```python
from build123d import *

# Parameters (mm, degrees)
SKETCH1_W                 = 75
SKETCH1_H                 = 40
BOSS_EXTRUDE1_DEPTH       = 8
SKETCH2_W                 = 72
SKETCH2_H                 = 17
SKETCH2_W_2               = 71
SKETCH2_H_2               = 16
CUT_EXTRUDE1_DEPTH        = 0.5
SKETCH3_W                 = 15
SKETCH3_H                 = 5
SKETCH3_W_2               = 7
SKETCH3_H_2               = 7
CUT_EXTRUDE3_DEPTH        = 3
DRAFT4_ANGLE              = 25
DRAFT5_ANGLE              = 25
DRAFT4_OF_MIRROR1_2_ANGLE = 25
DRAFT5_OF_MIRROR1_2_ANGLE = 25


with BuildPart() as part:
    # Sketch1 → Boss-Extrude1 (new body)
    with BuildSketch(Plane.XY):
        with Locations((37.5, 20)):
            Rectangle(SKETCH1_W, SKETCH1_H)
    extrude(amount=BOSS_EXTRUDE1_DEPTH)

    # Sketch2 → Cut-Extrude1 (cut)
    with BuildSketch(Plane.XY.offset(8)):
        with Locations((37.5, 10)):
            Rectangle(SKETCH2_W, SKETCH2_H)
        with Locations((37.5, 10)):
            Rectangle(SKETCH2_W_2, SKETCH2_H_2, mode=Mode.SUBTRACT)
    cut_extrude1 = extrude(amount=-CUT_EXTRUDE1_DEPTH, mode=Mode.SUBTRACT)

    # Sketch3 → Cut-Extrude3 (cut)
    with BuildSketch(Plane.XY.offset(8)):
        with Locations((37.5, 10)):
            Rectangle(SKETCH3_W, SKETCH3_H)
        with Locations((63.5, 10)):
            Rectangle(SKETCH3_W_2, SKETCH3_H_2)
    cut_extrude3 = extrude(amount=-CUT_EXTRUDE3_DEPTH, mode=Mode.SUBTRACT)

    # Draft4
    draft4_faces = [part.faces().sort_by_distance(p)[0] for p in [
        (45, 10, 6.5),
        (37.5, 7.5, 6.5),
        (30, 10, 6.5),
        (37.5, 12.5, 6.5),
    ]]
    draft(draft4_faces, Plane.XY.offset(8), DRAFT4_ANGLE)

    # Draft5
    draft5_faces = [part.faces().sort_by_distance(p)[0] for p in [
        (67, 10, 6.5),
        (63.5, 6.5, 6.5),
        (60, 10, 6.5),
        (63.5, 13.5, 6.5),
    ]]
    draft(draft5_faces, Plane.XY.offset(8), DRAFT5_ANGLE)

    # Sketch7 → Revolve2 (revolve)
    with BuildSketch(Plane(origin=(63.5, 0, 0), x_dir=(0, 0, -1), z_dir=(1, 0, 0)), mode=Mode.PRIVATE) as revolve2_sk:
        Polygon((-5, 10), (-5, 9.5), (-6.936491673, 10), align=None)
    revolve2 = revolve(revolve2_sk.sketch.rotate(Axis((63.5, 10, 6.936491673), (0, 0, -1)), 90), axis=Axis((63.5, 10, 6.936491673), (0, 0, -1)))

    # Mirror1: Cut-Extrude1, Cut-Extrude3, Revolve2 across plane
    add(cut_extrude1.mirror(Plane.ZX.offset(20)), mode=Mode.SUBTRACT)
    add(cut_extrude3.mirror(Plane.ZX.offset(20)), mode=Mode.SUBTRACT)
    add(revolve2.mirror(Plane.ZX.offset(20)))

    # Draft4 of Mirror1 2
    draft4_of_mirror1_2_faces = [part.faces().sort_by_distance(p)[0] for p in [
        (45, 30, 6.5),
        (37.5, 32.5, 6.5),
        (30, 30, 6.5),
        (37.5, 27.5, 6.5),
    ]]
    draft(draft4_of_mirror1_2_faces, Plane(origin=(0, 40, 8), x_dir=(1, 0, 0), z_dir=(0, 0, 1)), DRAFT4_OF_MIRROR1_2_ANGLE)

    # Draft5 of Mirror1 2
    draft5_of_mirror1_2_faces = [part.faces().sort_by_distance(p)[0] for p in [
        (67, 30, 6.5),
        (63.5, 33.5, 6.5),
        (60, 30, 6.5),
        (63.5, 26.5, 6.5),
    ]]
    draft(draft5_of_mirror1_2_faces, Plane(origin=(0, 40, 8), x_dir=(1, 0, 0), z_dir=(0, 0, 1)), DRAFT5_OF_MIRROR1_2_ANGLE)


solid = part.part
```
The model under review builds one solid part; all positions refer to its coordinate system, in mm. A direction names the side the tool comes from. Round coordinates to 2 decimals unless told otherwise and drop trailing zeros. Write each loop counter-clockwise with the first axis right and the second up, starting at its lowest first coordinate (ties: lowest second). Pieces come first, ordered by that corner, then holes. Notation, with made-up numbers: M -9.5,-32.5 L 47.5,-32.5 A18 cw 47.5,-4.5 Z; hole C 43,55.25 d7. An arc over 180 degrees is marked long. Use CSV: the item, a comma, the result in double quotes. Start each with the question number.
(1) The part is to be moulded in two halves that separate along Y. For faces 3 (the face through (0, 20, 4)), 4 (the face through (37, 40, 4)), 5 (the face through (37.3, 18.2, 7.5)), say which applies: +Y half, -Y half, draft (parallel to the pull), parting line (faces both ways), or undercut.
(2) For line 1 along X through (y, z) = (29.5, 6.75); line 2 along X through (y, z) = (11, 5.5); line 3 along Y through (x, z) = (34.5, 6), list the stretches that pass through material, from the lowest coordinate up.
(3) We need section A-A, the plane x = 37. State the section outline as (y, z) points.
(4) Clearance check with flat-ended pins moving along their axes: P1, Ø3.5, axis at x = 64, y = 11, coming from the +Z side; P2, Ø1.1, axis at x = 36, y = 30.5, coming from the +Z side. State where each tip first meets the part, or that it passes through.
(5) Tool access review of faces 1 (the face through (63.5, 12.8, 6.5)), 2 (the face through (37, 34, 8)): name each direction out of +Z, -Z, +X, -X, +Y, -Y from which nothing blocks a thin tool from reaching the whole face with its end or side.
Findings:
1,face 3,"draft"
1,face 4,"+Y half"
1,face 5,"undercut"
2,line 1,"0 to 30.58, 44.42 to 60.58, 66.42 to 75"
2,line 2,"0 to 31.17, 43.83 to 61.17, 65.83 to 75"
2,line 3,"0 to 8.43, 11.57 to 28.43, 31.57 to 40"
3,outline,"M 0,0 L 40,0 L 40,8 L 38.5,8 L 38.5,7.5 L 38,7.5 L 38,8 L 32.5,8 L 31.1,5 L 28.9,5 L 27.5,8 L 22,8 L 22,7.5 L 21.5,7.5 L 21.5,8 L 18.5,8 L 18.5,7.5 L 18,7.5 L 18,8 L 12.5,8 L 11.1,5 L 8.9,5 L 7.5,8 L 2,8 L 2,7.5 L 1.5,7.5 L 1.5,8 L 0,8 Z"
4,P1,"z = 6.94"
4,P2,"z = 5"
5,face 1,"+Z"
5,face 2,"+Z, +X, -X, +Y, -Y"
